Drawing for the job (mm, zero at the part's lowest x, y, z). Round coordinates to 2 decimals unless told otherwise and drop trailing zeros. Write each loop counter-clockwise with the first axis right and the second up, starting at its lowest first coordinate (ties: lowest second). Pieces come first, ordered by that corner, then holes. Notation, with made-up numbers: (44.5, 61) - (74.5, 61) arc R13 ccw to (74.5, 73) - close; hole circle Ø3 at (5.5, 77). An arc over 180 degrees is marked (long way). Answer in a Markdown table with one row per item.
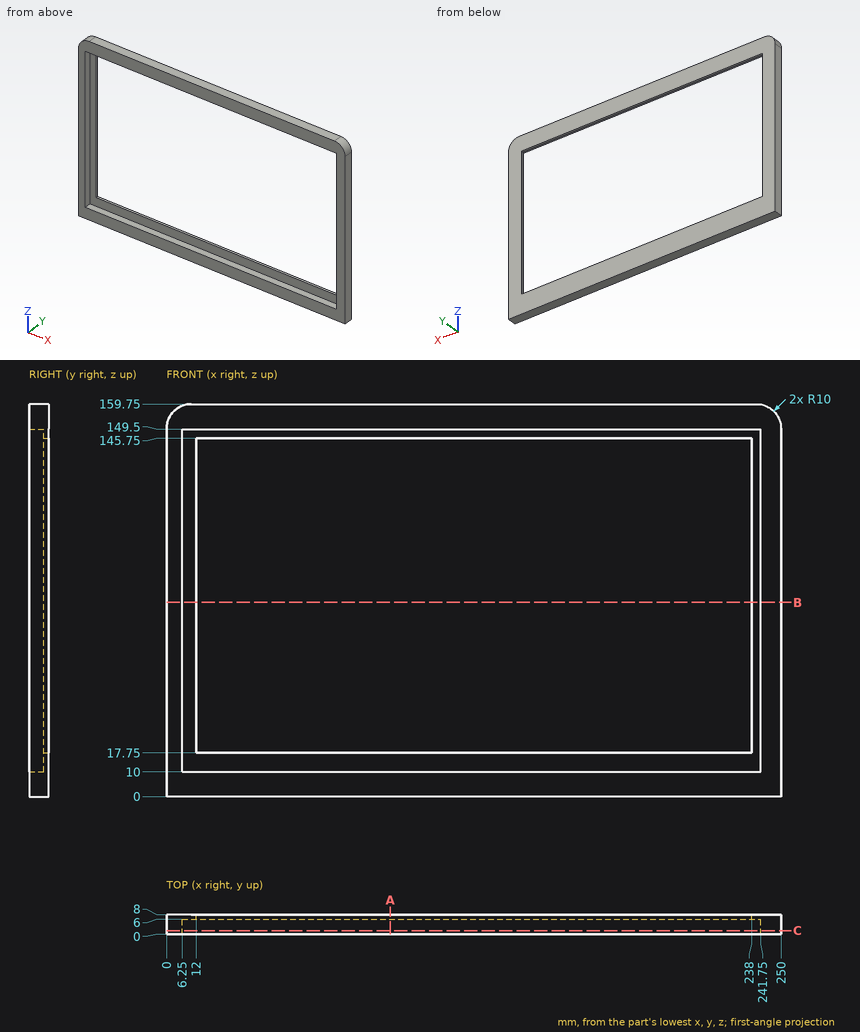
Q1. Drill centre lines: line 1 (X direction, y = 1.5, z = 107.5); line 2 (Z direction, x = 211.5, y = 5); line 3 (X direction, y = 6.5, z = 35.5). Where is each one in solid material? Low to high.
Computed:
| item | result |
|---|---|
| line 1 | x = 0 to 6.25, 241.75 to 250 |
| line 2 | z = 0 to 10, 149.5 to 159.75 |
| line 3 | x = 0 to 12, 238 to 250 |
Q2. Saw through at A-A on x = 91. List the corners of the cut face in (y, z), then the cut area to 3 significant figures.
Computed:
| item | result |
|---|---|
| outline | (0, 0) - (8, 0) - (8, 17.75) - (6, 17.75) - (6, 10) - (0, 10) - close; (0, 149.5) - (6, 149.5) - (6, 145.75) - (8, 145.75) - (8, 159.75) - (0, 159.75) - close |
| area | 185 mm2 |
Q3. Saw through at C-C on y = 1.5. List the corners of the cut face in (x, z), then the cut area to 3 significant figures.
Computed:
| item | result |
|---|---|
| outline | (0, 0) - (250, 0) - (250, 149.75) arc R10 ccw to (240, 159.75) - (10, 159.75) arc R10 ccw to (0, 149.75) - close; hole (6.25, 10) - (241.75, 10) - (241.75, 149.5) - (6.25, 149.5) - close |
| area | 7,040 mm2 |
Q4. Flat gauge pin, fed straight in: pin 1 (2 mm diameter, centred on x = 176.5, y = 6.5, fed in from -Z). Where does the tip first touch, or does it go through?
Computed:
| item | result |
|---|---|
| pin 1 | stops at z = 0 |
Q5. Saw through at B-B on z = 79. List the corners of the cut face in (x, y), then the cut area to 3 significant figures.
Computed:
| item | result |
|---|---|
| outline | (0, 0) - (6.25, 0) - (6.25, 6) - (12, 6) - (12, 8) - (0, 8) - close; (238, 6) - (241.75, 6) - (241.75, 0) - (250, 0) - (250, 8) - (238, 8) - close |
| area | 135 mm2 |
